from build123d import *

# Parameters (mm, degrees)
SKETCH2_R               = 20.6375
SKETCH2_R_2             = 15.875
BOSS_EXTRUDE1_DEPTH     = 9.525
CUT_EXTRUDE1_DEPTH      = 511.993168343
CUT_EXTRUDE1_DEPTH_BACK = 511.993168343


with BuildPart() as part:
    # Sketch1 → Revolve1 (revolve)
    with BuildSketch(Plane.XY, mode=Mode.PRIVATE) as revolve1_sk:
        with BuildLine():
            Line((-5.08, 17.526), (-500.634, 17.526))
            Line((-500.634, 17.526), (-500.634, 19.05))
            Line((-500.634, 19.05), (-5.08, 19.05))
            ThreePointArc((-5.08, 19.05), (-1.487897552, 17.562102448), (0, 13.97))
            Line((0, 13.97), (0, 11.176))
            Line((0, 11.176), (-1.524, 11.176))
            Line((-1.524, 11.176), (-1.524, 13.97))
            ThreePointArc((-1.524, 13.97), (-2.565528286, 16.484471714), (-5.08, 17.526))
        make_face()
    revolve(revolve1_sk.sketch.rotate(Axis((-484.828271433, 0, 0), (1, 0, 0)), 90), axis=Axis((-484.828271433, 0, 0), (1, 0, 0)))

    # Sketch2 → Boss-Extrude1 (add)
    with BuildSketch(Plane.ZY.offset(500.634)):
        with Locations(Location((0, 0, 0), (0, 0, 180))):
            Circle(SKETCH2_R)
        with Locations(Location((0, 0, 0), (0, 0, 180))):
            Circle(SKETCH2_R_2, mode=Mode.SUBTRACT)
    extrude(amount=BOSS_EXTRUDE1_DEPTH)

    # Sketch4 → Cut-Extrude1 (cut, two sides: drawn at the far end of the back side and taken through both)
    with BuildSketch(Plane.ZY.offset(510.159).offset(-CUT_EXTRUDE1_DEPTH_BACK)):
        with BuildLine():
            ThreePointArc((3.175, 20.391806719), (0, 20.6375), (-3.175, 20.391806719))
            ThreePointArc((-3.175, 20.391806719), (0, 19.277380448), (3.175, 20.391806719))
        make_face()
        with BuildLine():
            ThreePointArc((19.247322647, 7.446272702), (17.872599271, 10.31875), (16.072322647, 12.945534016))
            ThreePointArc((16.072322647, 12.945534016), (16.694701186, 9.638690224), (19.247322647, 7.446272702))
        make_face()
        with BuildLine():
            ThreePointArc((16.072322647, -12.945534016), (17.872599271, -10.31875), (19.247322647, -7.446272702))
            ThreePointArc((19.247322647, -7.446272702), (16.694701186, -9.638690224), (16.072322647, -12.945534016))
        make_face()
        with BuildLine():
            ThreePointArc((-3.175, -20.391806719), (0, -20.6375), (3.175, -20.391806719))
            ThreePointArc((3.175, -20.391806719), (0, -19.277380448), (-3.175, -20.391806719))
        make_face()
        with BuildLine():
            ThreePointArc((-19.247322647, -7.446272702), (-17.872599271, -10.31875), (-16.072322647, -12.945534016))
            ThreePointArc((-16.072322647, -12.945534016), (-16.694701186, -9.638690224), (-19.247322647, -7.446272702))
        make_face()
        with BuildLine():
            ThreePointArc((-16.072322647, 12.945534016), (-17.872599271, 10.31875), (-19.247322647, 7.446272702))
            ThreePointArc((-19.247322647, 7.446272702), (-16.694701186, 9.638690224), (-16.072322647, 12.945534016))
        make_face()
    extrude(amount=CUT_EXTRUDE1_DEPTH + CUT_EXTRUDE1_DEPTH_BACK, mode=Mode.SUBTRACT)


solid = part.part
The listing builds one solid part. Answer for the finished solid, in the listing's coordinates (mm). A direction names the side the tool comes from. Give positions to 0.01 mm unless a question says otherwise; leave off trailing zeros. Loops run counter-clockwise (first coordinate to the right, second up) from the corner with the lowest first, then second, coordinate; pieces in that order, holes last. Notation, with made-up numbers: (-20.5, -24.5) - (29.5, -24.5) arc R4 cw to (29.5, -17.5) - close; hole circle Ø7 at (36, 82.5). An arc over 180 degrees is marked (long way). Use one line per item in the form item = value.
1. Find the intervals of material crossed by line 1 along Z through (x, y) = (-437.5, -0.5); line 2 along Y through (x, z) = (-340, 11); line 3 along X through (y, z) = (10, -5.5), in increasing order. Write a range as [from, to].
Calculated:
line_1 = [-19.04, -17.52], [17.52, 19.04]
line_2 = [-15.55, -13.64], [13.64, 15.55]
line_3 = [-1.52, 0]
2. The mould has two halves that part along X. Classify faces 4 (the face through (-256.33, -5.26, 16.72)), 5 (the face through (-510.159, 12, 11)), 6 (the face through (-500.634, 13.5, 13.9)): pulls with the +X half, pulls with the -X half, needs draft (parallel to the pull), parting line crosses it, or undercut.
Calculated:
face_4 = undercut
face_5 = pulls with the -X half
face_6 = pulls with the +X half
3. Given pin 1 Ø10 at (x, y) = (-213, -1.5) entering from -Z; pin 2 Ø1 at (x, z) = (-97, 5) entering from -Y; pin 3 Ø12 at (x, y) = (-79.5, 13) entering from -Z; pin 4 Ø14 at (y, z) = (3, -1) entering from -X, each flat-ended and moving along its own axis, determine where each tip first touches the part or whether it passes through.
Calculated:
pin_1 = -19.05
pin_2 = -18.51
pin_3 = -17.72
pin_4 = through
4. Section B-B on x = -187.5 is taken. Give the vertices of the cut face in (y, z).
Calculated:
outline = circle Ø38.1 at (0, 0); hole circle Ø35.05 at (0, 0)
5. Which of the six approach directions +Z, -Z, +X, -X, +Y, -Y give full straight-line access (tool end or side, diameter ignored) to faces 1 (the face through (-249.388, 18.597, -4.13)), 2 (the face through (-1.524, -11.4, 0.1)), 3 (the face through (-500.634, -16, 3))?
Calculated:
face_1 = +X
face_2 = -X
face_3 = none
